```python
from build123d import *

# Parameters (mm, degrees)
F0_W     = 100
F0_H     = 40
F1_DEPTH = 10
F3_DEPTH = 10
F5_DEPTH = 305
F6_R     = 4.383557
F7_DEPTH = 345.001


with BuildPart() as f1:
    # F0 (on Top) → F1 (new body)
    with BuildSketch(Plane.XY):
        with Locations((50, 20)):
            Rectangle(F0_W, F0_H)
    extrude(amount=F1_DEPTH)

    # F2 (on face) → F3 (join)
    with BuildSketch(Plane.XZ):
        with BuildLine():
            Line((25.301725, 35), (25.301725, 0))
            Line((25.301725, 0), (74.698275, 0))
            Line((74.698275, 0), (74.698275, 35))
            ThreePointArc((74.698275, 35), (50, 59.698275), (25.301725, 35))
        make_face()
    extrude(amount=-F3_DEPTH)

    # F4 (on face) → F5 (join)
    with BuildSketch(Plane.XZ):
        with BuildLine():
            Line((0, 0), (25.301725, 0))
            Line((25.301725, 0), (25.301725, 3))
            Line((25.301725, 3), (74.698275, 3))
            Line((74.698275, 3), (74.698275, 0))
            Line((74.698275, 0), (100, 0))
            Line((100, 0), (100, 10))
            Line((100, 10), (74.698275, 10))
            Line((74.698275, 10), (74.698275, 35))
            ThreePointArc((74.698275, 35), (50, 59.698275), (25.301725, 35))
            Line((25.301725, 35), (25.301725, 10))
            Line((25.301725, 10), (0, 10))
            Line((0, 10), (0, 0))
        make_face()
    extrude(amount=F5_DEPTH)

    # F6 (on face) → F7 (cut, through all)
    with BuildSketch(Plane.XZ.offset(305)):
        with Locations((50.276015, 37.776016)):
            Circle(F6_R)
    extrude(amount=-F7_DEPTH, mode=Mode.SUBTRACT)


solid = f1.part
```
Verification items for the finished model (mm, model axes). A direction names the side the tool comes from. Round coordinates to 2 decimals unless told otherwise and drop trailing zeros. Write each loop counter-clockwise with the first axis right and the second up, starting at its lowest first coordinate (ties: lowest second). Pieces come first, ordered by that corner, then holes.
1. Section check B-B on y = -260. Enter the section's corners in (x, z), plus the area to 3 significant figures.
2. Access from +Z, -Z, +X, -X, +Y, -Y to the whole of each face (thin tool, end or side, straight path). Record for faces 4 (the flat face through (50, 10, 30)), 5 (the flat face through (25.302, -145, 23)), 6 (the flat face through (100, -135, 5)).
3. Section check D-D on z = 18.5. Enter the section's corners in (x, y).
4. Section check A-A on x = 50. Enter the section's corners in (y, z).
5. Section check C-C on x = 80. Enter the section's corners in (y, z).
6. Draft check along X on faces 1 (the flat face through (49, 40, 5)), 2 (the flat face through (50, -150, 3)), 3 (the flat face through (74.698, -145, 22)). Enter one of: +X half, -X half, draft (parallel to the pull), parting line (faces both ways), or undercut.
7. Scan lines: L1, parallel to Z at x = 50.5, y = -90; L2, parallel to Y at x = 62, z = 51; L3, parallel to X at y = -184, z = 11.5. Record each from-to range of solid material in increasing order.
8. Gauge pin test, flat ends, axial feed: P1, Ø3.5, axis at x = 41.5, z = 1, coming from the -Y side; P2, Ø20, axis at y = -151, z = 26, coming from the +X side; P3, Ø24.5, axis at x = 39, y = -100, coming from the -Z side; P4, Ø2.5, axis at y = -87, z = 1, coming from the -X side. Record the tip position at first contact, or that the pin passes through.
Answer:
1. outline: (0, 0) - (25.3, 0) - (25.3, 3) - (74.7, 3) - (74.7, 0) - (100, 0) - (100, 10) - (74.7, 10) - (74.7, 35) arc R24.7 ccw to (25.3, 35) - (25.3, 10) - (0, 10) - close; hole circle Ø8.77 at (50.28, 37.78)
1. area: 2,980 mm2
2. face 4: +Z, +X, -X, +Y
2. face 5: +Z, -X, +Y, -Y
2. face 6: +Z, -Z, +X, +Y, -Y
3. outline: (25.3, -305) - (74.7, -305) - (74.7, 10) - (25.3, 10) - close
4. outline: (-305, 3) - (0, 3) - (0, 0) - (40, 0) - (40, 10) - (10, 10) - (10, 33.4) - (-305, 33.4) - close; (-305, 42.15) - (10, 42.15) - (10, 59.7) - (-305, 59.7) - close
5. outline: (-305, 0) - (40, 0) - (40, 10) - (-305, 10) - close
6. face 1: draft
6. face 2: undercut
6. face 3: +X half
7. L1: z = 3 to 33.4, 42.15 to 59.69
7. L2: y = -305 to 10
7. L3: x = 25.3 to 74.7
8. P1: stops at y = 0
8. P2: stops at x = 74.7
8. P3: stops at z = 3
8. P4: stops at x = 0
